Geometry: final body of the model. Coordinates: model frame, mm. Give positions to 0.01 mm unless a question says otherwise; leave off trailing zeros. Order: outer loops, then holes, each group sorted by start corner. A loop starts at its lowest first (then second) coordinate and runs counter-clockwise, first axis right, second up. Notation, with made-up numbers: (89, 88) - (130, 88) arc R8 cw to (130, 100) - close; hole circle Ø10 at (52.25, 38). An arc over 180 degrees is marked (long way). One line per question, with ' | ' between items. Start each with the question number.
from build123d import *

# Parameters (mm, degrees)
SKETCH1_R           = 20
SKETCH1_R_2         = 14
BOSS_EXTRUDE1_DEPTH = 30
SKETCH2_R           = 20
SKETCH2_R_2         = 15
CUT_EXTRUDE1_DEPTH  = 20
FILLET1_R           = 10


with BuildPart() as part:
    # Sketch1 → Boss-Extrude1 (new body)
    with BuildSketch(Plane.XY):
        Circle(SKETCH1_R)
        Circle(SKETCH1_R_2, mode=Mode.SUBTRACT)
    extrude(amount=BOSS_EXTRUDE1_DEPTH)

    # Sketch2 → Cut-Extrude1 (cut)
    with BuildSketch(Plane(origin=(0, 0, 0), x_dir=(-1, 0, 0), z_dir=(0, 0, -1))):
        Circle(SKETCH2_R)
        Circle(SKETCH2_R_2, mode=Mode.SUBTRACT)
    extrude(amount=-CUT_EXTRUDE1_DEPTH, mode=Mode.SUBTRACT)

    # Fillet1
    # the kernel refuses this fillet: 10 mm, written as the material it adds along each edge
    with BuildSketch(Plane(origin=(0, 0, 20), x_dir=(-1, 0, 0), z_dir=(0, -1, 0))) as fillet1_piece_1:
        with BuildLine():
            CenterArc((25, 8.660254038), FILLET1_R, 180, 60)
            Line((20, 0), (19.9, -0.173205081))
            ThreePointArc((19.9, -0.173205081), (17.5, -0.2), (15, -0.2))
            Line((15, -0.2), (14.8, 0))
            Line((14.8, 0), (14.8, 8.660254038))
            Line((14.8, 8.660254038), (15, 8.660254038))
        make_face()
    revolve(axis=Axis((0, 0, 20), (0, 0, -1)))
    # the kernel refuses this fillet: 10 mm, written as the material it takes off along each edge
    with BuildSketch(Plane(origin=(0, 0, 0), x_dir=(-1, 0, 0), z_dir=(0, -1, 0))) as fillet1_2_piece_1:
        with BuildLine():
            CenterArc((5, -4.358898944), FILLET1_R, 0, 25.841932763)
            Line((14, 0), (14.18, 0.087177979))
            ThreePointArc((14.18, 0.087177979), (14.5, 0.2), (15, 0.2))
            Line((15, 0.2), (15.2, 0))
            Line((15.2, 0), (15.2, -4.358898944))
            Line((15.2, -4.358898944), (15, -4.358898944))
        make_face()
    revolve(axis=Axis((0, 0, 0), (0, 0, -1)), mode=Mode.SUBTRACT)


solid = part.part
(1) Material intervals for line 1 along X through (y, z) = (0, 22.5); line 2 along X through (y, z) = (2, 5), sorted ascending. Write a range as from..to.
(2) Cut plane B-B, the plane z = 26.5. Return the cut outline in (x, y), plus the area to 3 significant figures.
(3) Cut plane A-A, the plane z = 9.5. Return the cut outline in (x, y), plus the area to 3 significant figures.
(4) Pull-direction query (X, two-part tool) for faces 1 (the cylindrical face through (14.985, 0.66, 7.8)), 2 (the cylindrical face through (12.932, -5.362, 14.79)), 3 (the flat face through (-14, -4, 30)); classes: +X half, -X half, draft (parallel to the pull), parting line (faces both ways), or undercut.
(5) Contact query for flat-ended pins moving along their axis: P1, Ø10, axis at y = 13.5, z = 8.5, coming from the +X side; P2, Ø1.5, axis at x = 8.5, z = 24, coming from the +Y side; P3, Ø1, axis at x = 3, z = 23, coming from the +Y side. Output: stop coordinate, or through.
Results are:
1) line 1: -20..-14, 14..20 | line 2: -14.87..-13.86, 13.86..14.87
2) outline: circle Ø40 at (0, 0); hole circle Ø28 at (0, 0) | area: 641 mm2
3) outline: circle Ø30 at (0, 0); hole circle Ø28 at (0, 0) | area: 91.1 mm2
4) face 1: parting line | face 2: undercut | face 3: draft
5) P1: x = 12.36 | P2: y = 18.44 | P3: y = 19.84
